from build123d import *

# Parameters (mm, degrees)
SKETCH_1_W          = 6
SKETCH_1_H          = 12
EXTRUDE_1_DEPTH     = 70
SKETCH_2_W          = 16
SKETCH_2_H          = 12
EXTRUDE_2_DEPTH     = 3
SKETCH_3_R          = 1.65
CUT_EXTRUDE_1_DEPTH = 3
SKETCH_4_W          = 8
SKETCH_4_H          = 60
CUT_EXTRUDE_2_DEPTH = 3
CUT_EXTRUDE_3_DEPTH = 3


with BuildPart() as part:
    # 草图1 → 凸台-拉伸1 (new body)
    with BuildSketch(Plane(origin=(0, 0, 0), x_dir=(1, 0, 0), z_dir=(0, 1, 0))):
        Rectangle(SKETCH_1_W, SKETCH_1_H)
    extrude(amount=EXTRUDE_1_DEPTH)

    # 草图2 → 凸台-拉伸2 (add)
    with BuildSketch(Plane(origin=(0, 0, 0), x_dir=(1, 0, 0), z_dir=(0, 1, 0))):
        with Locations((-5, 0)):
            Rectangle(SKETCH_2_W, SKETCH_2_H)
    extrude(amount=-EXTRUDE_2_DEPTH)

    # 草图3 → 切除-拉伸1 (cut)
    with BuildSketch(Plane(origin=(0, 0, 0), x_dir=(1, 0, 0), z_dir=(0, 1, 0))):
        with Locations(Location((-8, 0, 0), (0, 0, 270))):
            Circle(SKETCH_3_R)
    extrude(amount=-CUT_EXTRUDE_1_DEPTH, mode=Mode.SUBTRACT)

    # 草图4 → 切除-拉伸2 (cut)
    with BuildSketch(Plane(origin=(-3, 0, 0), x_dir=(0, 0, -1), z_dir=(1, 0, 0))):
        with Locations((0, 40)):
            Rectangle(SKETCH_4_W, SKETCH_4_H)
    extrude(amount=CUT_EXTRUDE_2_DEPTH, mode=Mode.SUBTRACT)

    # 草图5 → 切除-拉伸3 (cut)
    with BuildSketch(Plane.ZY):
        with BuildLine():
            Line((1.65, 65), (1.65, 15))
            ThreePointArc((1.65, 15), (0, 13.35), (-1.65, 15))
            Line((-1.65, 15), (-1.65, 65))
            ThreePointArc((-1.65, 65), (0, 66.65), (1.65, 65))
        make_face()
    extrude(amount=-CUT_EXTRUDE_3_DEPTH, mode=Mode.SUBTRACT)


solid = part.part
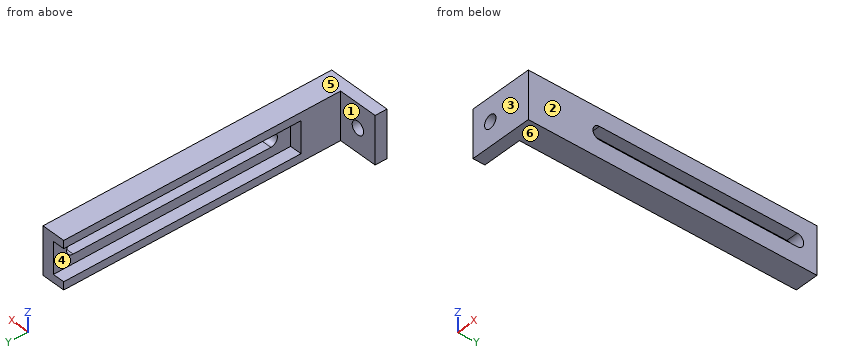
Read the model definition and answer for the solid it produces. Units are mm, in the model's axes. Face numbers are marked on the shaded views. A direction names the side the tool comes from. Coordinates: 2 decimals unless noted, no trailing zeros. Order: outer loops, then holes, each group sorted by start corner. A loop starts at its lowest first (then second) coordinate and runs counter-clockwise, first axis right, second up. Notation, with made-up numbers: (-4, -33) -> (20, -33) arc R18 cw to (20, -24) -> close; hole circle Ø9 at (-28.5, 43.25). An arc over 180 degrees is marked (long way). Answer as a JSON object with one key per item and string values.
1) The mould has two halves that part along Z. Classify the marked faces 3, 4, 5 and 6: released by +Z, released by -Z, zero draft, split by the parting line, or undercut.
Model answer:
{"face 3": "zero draft", "face 4": "undercut", "face 5": "released by +Z", "face 6": "released by -Z"}
2) A cutting plane is placed at A-A, the plane z = 0. Determine the outline of the cut face in (x, y).
Model answer:
{"outline": "(-13, -3) -> (-9.65, -3) -> (-9.65, 0) -> (-13, 0) -> close; (-6.35, -3) -> (3, -3) -> (3, 13.35) -> (0, 13.35) -> (0, 10) -> (-3, 10) -> (-3, 0) -> (-6.35, 0) -> close; (0, 66.65) -> (3, 66.65) -> (3, 70) -> (0, 70) -> close"}
3) Consider line 1 along X through (y, z) = (-1.95, 0); line 2 along Y through (x, z) = (-6.75, 5); line 3 along X through (y, z) = (35.5, 4.5). Determine where each line is inside the solid, lowest interval first. Write a range as from..to.
Model answer:
{"line 1": "x = -13..-9.65, -6.35..3", "line 2": "y = -3..0", "line 3": "x = -3..3"}
4) A cutting plane is placed at D-D, the plane z = -3. Determine the outline of the cut face in (x, y), plus the area to 3 significant figures.
Model answer:
{"outline": "(-13, -3) -> (3, -3) -> (3, 70) -> (0, 70) -> (0, 10) -> (-3, 10) -> (-3, 0) -> (-13, 0) -> close", "area": "288 mm²"}
5) A cutting plane is placed at C-C, the plane x = -8. Determine the outline of the cut face in (y, z).
Model answer:
{"outline": "(-3, -6) -> (0, -6) -> (0, -1.65) -> (-3, -1.65) -> close; (-3, 1.65) -> (0, 1.65) -> (0, 6) -> (-3, 6) -> close"}
6) Each of these flat-tipped pins is pushed along its axis until it touches: pin 1 (5 mm diameter, centred on y = 38.5, z = 4.5, fed in from -X); pin 2 (1.5 mm diameter, centred on y = 29.5, z = -2, fed in from -X); pin 3 (5 mm diameter, centred on x = -1, z = 3, fed in from +Y); pin 4 (3.5 mm diameter, centred on x = -2, z = -0.5, fed in from +Y). Where does it stop, or does it pass through?
Model answer:
{"pin 1": "stops at x = -3", "pin 2": "stops at x = 0", "pin 3": "stops at y = 70", "pin 4": "stops at y = 10"}
7) A cutting plane is placed at B-B, the plane y = 39. Determine the outline of the cut face in (x, z), plus the area to 3 significant figures.
Model answer:
{"outline": "(-3, -6) -> (3, -6) -> (3, -1.65) -> (0, -1.65) -> (0, -4) -> (-3, -4) -> close; (-3, 4) -> (0, 4) -> (0, 1.65) -> (3, 1.65) -> (3, 6) -> (-3, 6) -> close", "area": "38.1 mm²"}
8) A tool of negligible diameter and unlimited length cuts with its end or side. For the marked faces 1 and 2, from which of +Z, -Z, +X, -X, +Y, -Y can it reach the whole face along a straight path? Write none if from no direction.
Model answer:
{"face 1": "+Z, -Z, -X, +Y", "face 2": "+Z, -Z, +X, +Y, -Y"}
